```python
from build123d import *

# Parameters (mm, degrees)
F0_W     = 30
F0_H     = 20
F0_W_2   = 69.394279
F1_DEPTH = 30
F2_R     = 20


with BuildPart() as f1:
    # F0 (on Front) → F1 (new body)
    with BuildSketch(Plane.XZ):
        Polygon((159.634272, 0), (9.634272, -370), (59.634272, -370), (359.634272, -52.857143), (380.282107, -31.029432), (359.634272, -9.20172), (359.634272, 0), (419.442074, 58.0528), (425.315722, 52.496647), (438.374084, 30.382087), (459.824098, 53.057817), (759.634272, 370), (690.239993, 370), (690.239993, 340), (459.984443, 96.58699), (432.284971, 204.239834), (502.989308, 340), (475.40856, 340), (424.809358, 233.293495), (401.886582, 340), (389.634272, 370), (359.634272, 370), (-10.365728, 370), (-40.365728, 370), align=None)
        Polygon((173.899783, -26.391195), (194.902527, 0), (416.868696, 131.068154), (124.228867, -273.426068), (80.174812, -270), align=None, mode=Mode.SUBTRACT)
        Polygon((165.477519, 52.279216), (6.237836, 340), (341.3015, 340), align=None, mode=Mode.SUBTRACT)
        Polygon((179.74303, 25.888021), (371.932986, 338.332056), (404.63926, 158.686339), align=None, mode=Mode.SUBTRACT)
        Polygon((490.629017, 373.237222), (474.996572, 340), (475.40856, 340), (502.989308, 340), (519.577146, 371.850489), align=None)
        Polygon((490.629017, 390), (490.629017, 373.237222), (519.577146, 371.850489), (519.577146, 390), align=None)
        with Locations((374.634272, 380)):
            Rectangle(F0_W, F0_H)
        with Locations((724.937132, 380)):
            Rectangle(F0_W_2, F0_H)
        with Locations((-25.365728, 380)):
            Rectangle(F0_W, F0_H)
        Polygon((380.282107, -31.029432), (359.634272, -52.857143), (659.634272, -370), (709.634272, -370), (459.824098, 53.057817), (438.374084, 30.382087), (617.768873, -273.426068), (546.664514, -206.919405), align=None)
        Polygon((359.634272, -9.20172), (380.282107, -31.029432), (438.374084, 30.382087), (425.315722, 52.496647), (419.442074, 58.0528), (359.634272, 0), align=None)
    extrude(amount=F1_DEPTH)

    # F2
    f2_edges = [f1.edges().sort_by_distance(p)[0] for p in [
        (173.899783, -15, -26.391195),
        (194.902527, -15, 0),
        (416.868696, -15, 131.068154),
        (124.228867, -15, -273.426068),
        (80.174812, -15, -270),
        (179.74303, -15, 25.888021),
        (432.284971, -15, 204.239834),
        (459.984443, -15, 96.58699),
        (424.809358, -15, 233.293495),
        (371.932986, -15, 338.332056),
        (165.477519, -15, 52.279216),
        (6.237836, -15, 340),
        (341.3015, -15, 340),
        (404.63926, -15, 158.686339),
        (617.768873, -15, -273.426068),
        (438.374084, -15, 30.382087),
        (380.282107, -15, -31.029432),
        (359.634272, -15, -52.857143),
        (459.824098, -15, 53.057817),
        (401.886582, -15, 340),
        (389.634272, -15, 370),
    ]]
    fillet(f2_edges, radius=F2_R)


solid = f1.part
```
Check sheet for the modelled part. Datum: model origin and axes. Units: mm. A direction names the side the tool comes from. Coordinates: 2 decimals unless noted, no trailing zeros. Write each loop counter-clockwise with the first axis right and the second up, starting at its lowest first coordinate (ties: lowest second). Pieces come first, ordered by that corner, then holes. Notation, with made-up numbers: (10, 80.25) -> (28, 80.25) arc R12 ccw to (28, 96.25) -> close; hole circle Ø11 at (62.25, -1.5). An arc over 180 degrees is marked (long way). Use a Markdown table: item, result.
1. Tool access check on faces 4 (the flat face through (462.91, -14.79, 313.64)), 5 (the flat face through (612.88, -14.79, 214.86)), 6 (the flat face through (514.901, -14.79, -216.996)), 7 (the flat face through (86.634, -14.79, 194.737)). Record the directions out of +Z, -Z, +X, -X, +Y, -Y that give a thin tool (end or side, any length) a straight path to the whole face; none if there is none.
Reported:
| item | result |
|---|---|
| face 4 | +Z, +Y, -Y |
| face 5 | +X, +Y, -Y |
| face 6 | -Z, +Y, -Y |
| face 7 | +Y, -Y |
2. Sectioned sample at C-C (y = -18). Give the number of separate pieces and of enclosed holes in the cut face, plus the area to 3 significant figures.
Reported:
| item | result |
|---|---|
| separate pieces | 1 |
| enclosed holes | 4 |
| area | 144,000 mm2 |
3. Scan lines: line 1 along Z through (x, y) = (58.5, -28); line 2 along X through (y, z) = (-29, -141.5); line 3 along Z through (x, y) = (483, -25.5). Record each from-to range of solid material in increasing order.
Reported:
| item | result |
|---|---|
| line 1 | z = -370 to -249.46, 187.1 to 245.57, 340 to 370 |
| line 2 | x = 102.27 to 129.61, 219.67 to 275.78, 443.49 to 484.78, 539.87 to 574.71 |
| line 3 | z = -183.27 to -139.62, -45.19 to 13.81, 77.56 to 121.15, 301.62 to 357.02 |
4. Release check for a two-part mould opening along X. For faces 1 (the cylindrical face through (323.23, -15.21, 329.52)), 2 (the cylindrical face through (464.81, -15.21, 52.31)), 3 (the cylindrical face through (91.42, -15.21, -262.59)) record: pulls with the +X half, pulls with the -X half, needs draft (parallel to the pull), parting line crosses it, or undercut.
Reported:
| item | result |
|---|---|
| face 1 | undercut |
| face 2 | pulls with the +X half |
| face 3 | undercut |
5. Sectioned sample at B-B (x = 647). Enter the section's corners in (y, z), plus the area to 3 significant figures.
Reported:
| item | result |
|---|---|
| outline | (-30, -356.64) -> (0, -356.64) -> (0, -263.93) -> (-30, -263.93) -> close; (-30, 250.93) -> (0, 250.93) -> (0, 294.29) -> (-30, 294.29) -> close |
| area | 4,080 mm2 |
6. Sectioned sample at A-A (z = 253). Enter the section's corners in (x, y), plus the area to 3 significant figures.
Reported:
| item | result |
|---|---|
| outline | (22.88, -30) -> (54.39, -30) -> (54.39, 0) -> (22.88, 0) -> close; (288.14, -30) -> (319.44, -30) -> (319.44, 0) -> (288.14, 0) -> close; (387.47, -30) -> (457.68, -30) -> (457.68, 0) -> (387.47, 0) -> close; (607.94, -30) -> (648.96, -30) -> (648.96, 0) -> (607.94, 0) -> close |
| area | 5,220 mm2 |
7. Sectioned sample at D-D (z = -288.5). Enter the section's corners in (x, y).
Reported:
| item | result |
|---|---|
| outline | (42.67, -30) -> (136.73, -30) -> (136.73, 0) -> (42.67, 0) -> close; (582.54, -30) -> (661.51, -30) -> (661.51, 0) -> (582.54, 0) -> close |
8. Go/stop test with flat-tipped pins: pin 1 Ø9 at (x, y) = (247, -18) entering from +Z; pin 2 Ø2 at (x, y) = (152, -7.5) entering from -Z; pin 3 Ø10 at (y, z) = (-10, -13) entering from -X. Record where each tip stops, or that it passes through.
Reported:
| item | result |
|---|---|
| pin 1 | stops at z = 370 |
| pin 2 | stops at z = -273.41 |
| pin 3 | stops at x = 152.34 |
